Geometry check sheet. Reference: the model listing, model coordinates, mm. Coordinates: 2 decimals unless noted, no trailing zeros. Order: outer loops, then holes, each group sorted by start corner. A loop starts at its lowest first (then second) coordinate and runs counter-clockwise, first axis right, second up.
```python
from build123d import *

# Parameters (mm, degrees)
F0_R     = 4.5
F0_R_2   = 25.025
F1_DEPTH = 10


with BuildPart() as f1:
    # F0 (on Front) → F1 (new body)
    with BuildSketch(Plane.XZ):
        with BuildLine():
            ThreePointArc((-33, 37), (-41.485281, 33.485281), (-45, 25))
            Line((-45, 25), (-45, -25))
            ThreePointArc((-45, -25), (-41.485281, -33.485281), (-33, -37))
            Line((-33, -37), (33, -37))
            ThreePointArc((33, -37), (41.485281, -33.485281), (45, -25))
            Line((45, -25), (45, 25))
            ThreePointArc((45, 25), (41.485281, 33.485281), (33, 37))
            Line((33, 37), (-33, 37))
        make_face()
        with Locations((-33, -25)):
            Circle(F0_R, mode=Mode.SUBTRACT)
        with Locations((33, -25)):
            Circle(F0_R, mode=Mode.SUBTRACT)
        with Locations((-33, 25)):
            Circle(F0_R, mode=Mode.SUBTRACT)
        Circle(F0_R_2, mode=Mode.SUBTRACT)
        with Locations((33, 25)):
            Circle(F0_R, mode=Mode.SUBTRACT)
    extrude(amount=F1_DEPTH)


solid = f1.part
```
Item 1: Sectioned sample at A-A (z = 0). Record the cut outline in (x, y) (3 decimals).
Item 2: Release check for a two-part mould opening along Z. For faces 1 (the face through (-30.581, -4.93, -21.206)), 2 (the face through (41.39, -4.93, -33.58)), 3 (the face through (41.58, -4.93, 33.39)) record: pulls with the +Z half, pulls with the -Z half, needs draft (parallel to the pull), parting line crosses it, or undercut.
Item 3: Sectioned sample at B-B (x = 0). Record the cut outline in (y, z) (3 decimals), and give its area (4 significant figures).
Item 4: Thickness scan on line 1 along Z through (x, y) = (33, -3.75); line 2 along X through (y, z) = (-1.25, 21); line 3 along X through (y, z) = (-4.25, 26). Record the ranges inside material, lowest first.
Item 5: Sectioned sample at D-D (z = 28.5). Record the cut outline in (x, y), and give its area (3 significant figures).
Item 6: Sectioned sample at C-C (y = -4). Record the cut outline in (x, z) (3 decimals).
Geometry check:
1. outline: (-45, -10) - (-25.025, -10) - (-25.025, 0) - (-45, 0) - close; (25.025, -10) - (45, -10) - (45, 0) - (25.025, 0) - close
2. face 1: undercut
2. face 2: pulls with the -Z half
2. face 3: pulls with the +Z half
3. outline: (-10, -37) - (0, -37) - (0, -25.025) - (-10, -25.025) - close; (-10, 25.025) - (0, 25.025) - (0, 37) - (-10, 37) - close
3. area: 239.5 mm2
4. line 1: z = -37 to -29.5, -20.5 to 20.5, 29.5 to 37
4. line 2: x = -45 to -35.06, -30.94 to -13.61, 13.61 to 30.94, 35.06 to 45
4. line 3: x = -44.96 to -37.39, -28.61 to 28.61, 37.39 to 44.96
5. outline: (-44.48, -10) - (-35.83, -10) - (-35.83, 0) - (-44.48, 0) - close; (-30.17, -10) - (30.17, -10) - (30.17, 0) - (-30.17, 0) - close; (35.83, -10) - (44.48, -10) - (44.48, 0) - (35.83, 0) - close
5. area: 776 mm2
6. outline: (-45, -25) arc R12 ccw to (-33, -37) - (33, -37) arc R12 ccw to (45, -25) - (45, 25) arc R12 ccw to (33, 37) - (-33, 37) arc R12 ccw to (-45, 25) - close; hole circle Ø9 at (-33, -25); hole circle Ø9 at (-33, 25); hole circle Ø50.05 at (0, 0); hole circle Ø9 at (33, -25); hole circle Ø9 at (33, 25)
